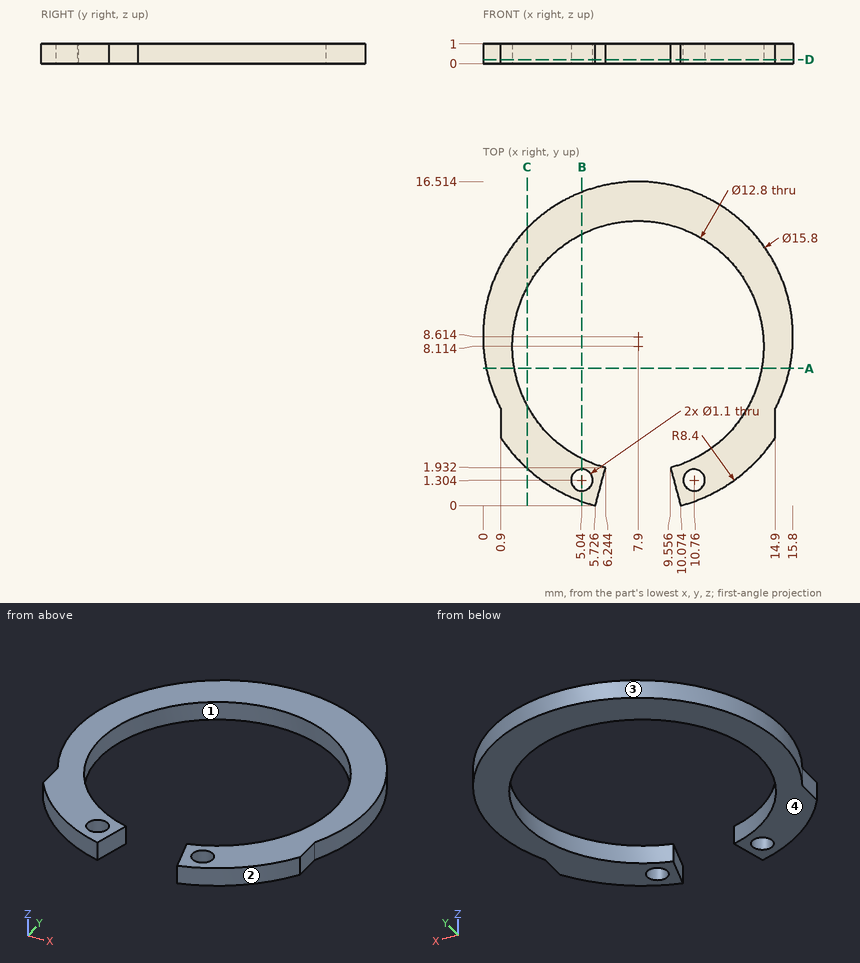
Answer from the drawing. Dimensions are ordinates in mm from the lowest x, y and z of the part. Round coordinates to 2 decimals unless told otherwise and drop trailing zeros. Order: outer loops, then holes, each group sorted by start corner. A loop starts at its lowest first (then second) coordinate and runs counter-clockwise, first axis right, second up.
1) Straight lines are drawn through the part: L1, parallel to Y at x = 5.04, z = 0.45 (1 decimal); L2, parallel to Y at x = 4.75, z = 0.9 (1 decimal); L3, parallel to X at y = 4.75, z = 0.6 (1 decimal). For each, find the intervals that lie inside material, in ascending order.
2) A flat-ended cylindrical pin translates along its axis: pin 1 (0.5 mm diameter, centred on y = 4.5, z = 0.5, fed in from -X). Find the tip coordinate at first contact, or state that the pin passes through.
3) The part is cut by section D-D on z = 0.2. Write down the section's boundary in (x, y).
4) The part is cut by section A-A on y = 7. Write down the section's boundary in (x, z).
5) The mould has two halves that part along X. Classify the marked faces 1, 2, 3 and 4: released by +X, released by -X, zero draft, split by the parting line, or undercut.
6) The part is cut by section B-B on x = 5.04. Write down the section's boundary in (y, z) (1 decimal).
7) The part is cut by section C-C on x = 2.25. Write down the section's boundary in (y, z) (1 decimal).
Resolved:
1. L1: y = 0.2 to 0.8, 1.9 to 2.4, 13.8 to 16
1. L2: y = 0.3 to 0.8, 1.8 to 2.5, 13.7 to 15.9
1. L3: x = 0.9 to 2.5, 13.3 to 14.9
2. pin 1: stops at x = 0.9
3. outline: (0.9, 3.47) arc R8.4 ccw to (5.73, 0) - (6.24, 1.93) arc R6.4 cw (long way) to (9.56, 1.93) - (10.07, 0) arc R8.4 ccw to (14.9, 3.47) - (14.9, 4.95) arc R7.9 ccw (long way) to (0.9, 4.95) - close; hole circle Ø1.1 at (5.04, 1.3); hole circle Ø1.1 at (10.76, 1.3)
4. outline: (0.17, 0) - (1.6, 0) - (1.6, 1) - (0.17, 1) - close; (14.2, 0) - (15.63, 0) - (15.63, 1) - (14.2, 1) - close
5. face 1: undercut
5. face 2: released by +X
5. face 3: split by the parting line
5. face 4: zero draft
6. outline: (0.2, 0) - (0.8, 0) - (0.8, 1) - (0.2, 1) - close; (1.9, 0) - (2.4, 0) - (2.4, 1) - (1.9, 1) - close; (13.8, 0) - (16, 0) - (16, 1) - (13.8, 1) - close
7. outline: (1.9, 0) - (5.1, 0) - (5.1, 1) - (1.9, 1) - close; (11.1, 0) - (14.1, 0) - (14.1, 1) - (11.1, 1) - close
